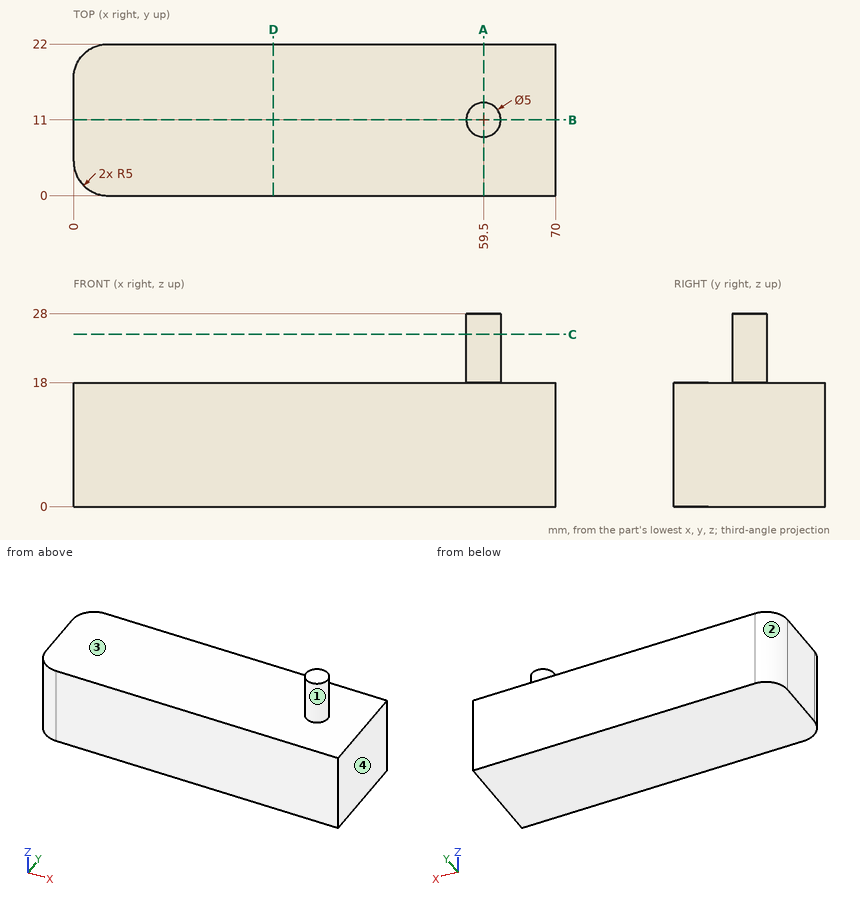
The drawing under review shows one solid part. Ordinate dimensions are in mm from its lowest x, y, z. Round coordinates to 2 decimals unless told otherwise and drop trailing zeros. Write each loop counter-clockwise with the first axis right and the second up, starting at its lowest first coordinate (ties: lowest second). Pieces come first, ordered by that corner, then holes.
(1) We need section A-A on x = 59.5. Give the boundary of the cut face in (y, z).
(2) We need section C-C on z = 25. Give the boundary of the cut face in (x, y), and give its area (3 significant figures).
(3) Insertion check: pin 1 (12 mm diameter, centred on x = 33.5, y = 10, fed in from +Z). The pin has a flat end and moves straight along its axis. Give the tip position at first contact, or say it passes through.
(4) We need section B-B on y = 11. Give the boundary of the cut face in (x, z).
(5) Mouldability with a two-part tool opening along X and no side actions: class the marked faces 1, 2, 3 and 4 as +X half, -X half, draft (parallel to the pull), parting line (faces both ways), or undercut.
(6) Wall thickness on L1, parallel to Z at x = 31, y = 10.25; L2, parallel to X at y = 18, z = 6.75; L3, parallel to X at y = 4.5, z = 1: over which ranges is each line inside the solid? List them lowest first.
(7) We need section D-D on x = 29. Give the boundary of the cut face in (y, z), and give its area (3 significant figures).
Findings below:
1. outline: (0, 0) - (22, 0) - (22, 18) - (13.5, 18) - (13.5, 28) - (8.5, 28) - (8.5, 18) - (0, 18) - close
2. outline: circle Ø5 at (59.5, 11)
2. area: 19.6 mm2
3. pin 1: stops at z = 18
4. outline: (0, 0) - (70, 0) - (70, 18) - (62, 18) - (62, 28) - (57, 28) - (57, 18) - (0, 18) - close
5. face 1: parting line
5. face 2: -X half
5. face 3: draft
5. face 4: +X half
6. L1: z = 0 to 18
6. L2: x = 0.1 to 70
6. L3: x = 0.03 to 70
7. outline: (0, 0) - (22, 0) - (22, 18) - (0, 18) - close
7. area: 396 mm2
